The model under review builds one solid part; all positions refer to its coordinate system, in mm. Face numbers are marked on the shaded views. A direction names the side the tool comes from. Give positions to 0.01 mm unless a question says otherwise; leave off trailing zeros. Loops run counter-clockwise (first coordinate to the right, second up) from the corner with the lowest first, then second, coordinate; pieces in that order, holes last. Notation, with made-up numbers: M 69.25,44 L 112.25,44 A21 ccw 112.25,51 Z; hole C -32,46.25 d7. An arc over 180 degrees is marked long. Return JSON: item names as keys, results as strings. Group by question number.
```python
from build123d import *

# Parameters (mm, degrees)
F0_W      = 17
F0_H      = 100
F1_DEPTH  = 1.5
F3_D      = 2.5
F4_W      = 1.5
F4_H      = 7.62
F5_ANGLE  = 90
F6_W      = 1.5
F6_H      = 7.62
F7_DEPTH  = 15
F9_D      = 2.5
F10_W     = 1.5
F10_H     = 9
F11_DEPTH = 1.501


with BuildPart() as f1:
    # F0 (on Front) → F1 (new body)
    with BuildSketch(Plane.XZ):
        with Locations((8.5, 50)):
            Rectangle(F0_W, F0_H)
    extrude(amount=F1_DEPTH)

    # F3 (through all)
    with Locations(Plane.XZ.offset(1.5)):
        with Locations((8.5, 96), (8.5, 4)):
            Hole(F3_D / 2)

    # F4 (on face) → F5 (revolve)
    with BuildSketch(Plane.YZ.offset(17)):
        with Locations((-0.75, 96.19)):
            Rectangle(F4_W, F4_H)
        with Locations((-0.75, 3.81)):
            Rectangle(F4_W, F4_H)
    revolve(axis=Axis((17, 0, 50), (0, 0, 1)), revolution_arc=F5_ANGLE)

    # F6 (on face) → F7 (join)
    with BuildSketch(Plane(origin=(0, 0, 0), x_dir=(-1, 0, 0), z_dir=(0, 1, 0))):
        with Locations((-17.75, 3.81)):
            Rectangle(F6_W, F6_H)
        with Locations((-17.75, 96.19)):
            Rectangle(F6_W, F6_H)
    extrude(amount=F7_DEPTH)

    # F9 (through all)
    with Locations(Plane(origin=(17, 0, 0), x_dir=(0, -1, 0), z_dir=(-1, 0, 0))):
        with Locations((-4.5145543722, 96.19), (-4.5145543722, 3.81)):
            Hole(F9_D / 2)

    # F10 (on face) → F11 (cut, through all)
    with BuildSketch(Plane(origin=(0, 0, 0), x_dir=(-1, 0, 0), z_dir=(0, 1, 0))):
        with Locations((-0.75, 95.5)):
            Rectangle(F10_W, F10_H)
        with Locations((-0.75, 4.5)):
            Rectangle(F10_W, F10_H)
    extrude(amount=-F11_DEPTH, mode=Mode.SUBTRACT)


solid = f1.part
```
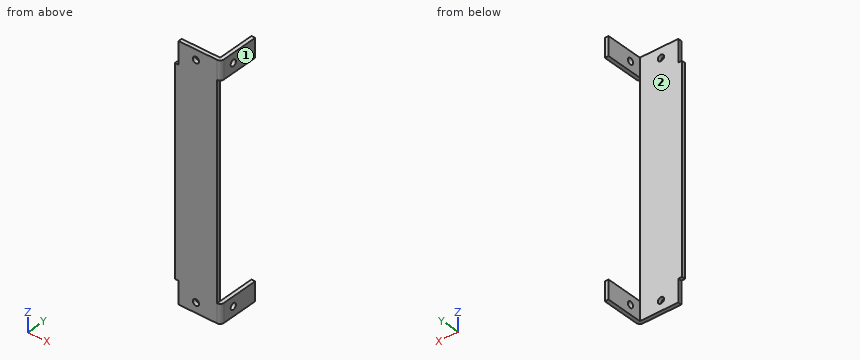
(1) For probe 1 along Z at (x, y) = (8.5, -0.5); probe 2 along Z at (x, y) = (17.5, 9); probe 3 along Y at (x, z) = (7.75, 43), list the stretches that pass through material, from the lowest coordinate up.
(2) Add section C-C (z = 52). Write out the cut boundary in (x, y), and give its area (3 significant figures).
(3) For the marked faces 1 and 2, list the 3-axis set-ups (+Z, -Z, +X, -X, +Y, -Y) from which the entire face can be reached by the end or side of a thin tool; tool diameter is ignored.
(4) For pin 1 (6 mm diameter, centred on y = 6, z = 97.5, fed in from -X); pin 2 (4 mm diameter, centred on x = 6, y = 0.5, fed in from -Z); pin 3 (0.8 mm diameter, centred on y = -0.5, z = 5, fed in from -X); pin 4 (2 mm diameter, centred on x = 4, z = 21, fed in from +Y), all flat-tipped, find the tip position at first contact; note any pin that passes through.
(5) Add section A-A (y = 11.5). Write out the cut boundary in (x, z), and give its area (3 significant figures).
(6) Add section B-B (x = 8.5). Write out the cut boundary in (y, z), and give its area (4 significant figures).
(7) Add section D-D (x = 2.5). Write out the cut boundary in (y, z), and give its area (3 significant figures).
Verdict:
{
 "1": {"probe 1": "z = 0 to 2.75, 5.25 to 94.75, 97.25 to 100", "probe 2": "z = 0 to 7.62, 92.38 to 100", "probe 3": "y = -1.5 to 0"},
 "2": {"outline": "M 0,-1.5 L 17,-1.5 L 17,0 L 0,0 Z", "area": "25.5 mm²"},
 "3": {"face 1": "+Z, -Z, +X, +Y, -Y", "face 2": "+Z, -Z, -X, +Y"},
 "4": {"pin 1": "stops at x = 17", "pin 2": "stops at z = 0", "pin 3": "stops at x = 1.5", "pin 4": "stops at y = 0"},
 "5": {"outline": "M 17,0 L 18.5,0 L 18.5,7.62 L 17,7.62 Z; M 17,92.38 L 18.5,92.38 L 18.5,100 L 17,100 Z", "area": "22.9 mm²"},
 "6": {"outline": "M -1.5,0 L 0,0 L 0,2.75 L -1.5,2.75 Z; M -1.5,5.25 L 0,5.25 L 0,94.75 L -1.5,94.75 Z; M -1.5,97.25 L 0,97.25 L 0,100 L -1.5,100 Z", "area": "142.5 mm²"},
 "7": {"outline": "M -1.5,0 L 0,0 L 0,100 L -1.5,100 Z", "area": "150 mm²"}
}
